For this review, take the finished solid that the model builds, in its own axes (mm). A direction names the side the tool comes from. Coordinates: 2 decimals unless noted, no trailing zeros. Order: outer loops, then holes, each group sorted by start corner. A loop starts at its lowest first (then second) coordinate and runs counter-clockwise, first axis right, second up.
from build123d import *

# Parameters (mm, degrees)
SKETCH1_R          = 8.5
SKETCH1_R_2        = 1.5
BASE_FLANGE1_DEPTH = 3


# Sheet-metal steps are written as plain solids
with BuildPart() as part:
    # Sketch1 → Base-Flange1 (new body)
    with BuildSketch(Plane(origin=(0, 0, 0), x_dir=(1, 0, 0), z_dir=(0, 1, 0))):
        with BuildLine():
            Line((19.609421573, -14.059417906), (10.862109445, -29.480175346))
            ThreePointArc((10.862109445, -29.480175346), (9.762567662, -30.59234701), (8.252687872, -31))
            Line((8.252687872, -31), (-8.352599575, -31))
            ThreePointArc((-8.352599575, -31), (-9.796606082, -30.629609326), (-10.884048227, -29.609896806))
            Line((-10.884048227, -29.609896806), (-20.742852548, -14.107625594))
            ThreePointArc((-20.742852548, -14.107625594), (-21.091885276, -13.336076582), (-21.211403896, -12.497728788))
            Line((-21.211403896, -12.497728788), (-21.211403896, 14.839305313))
            ThreePointArc((-21.211403896, 14.839305313), (-21.044943633, 15.824725306), (-20.564035521, 16.700789784))
            Line((-20.564035521, 16.700789784), (-10.150833328, 29.861484472))
            ThreePointArc((-10.150833328, 29.861484472), (-9.105019706, 30.700412322), (-7.798201703, 31))
            Line((-7.798201703, 31), (7.702138241, 31))
            ThreePointArc((7.702138241, 31), (9.077698333, 30.666052219), (10.147014932, 29.738556288))
            Line((10.147014932, 29.738556288), (19.444876691, 16.663267527))
            ThreePointArc((19.444876691, 16.663267527), (19.857851472, 15.837226972), (20, 14.924711239))
            Line((20, 14.924711239), (20, -12.57924256))
            ThreePointArc((20, -12.57924256), (19.900712388, -13.344662472), (19.609421573, -14.059417906))
        make_face()
        with Locations(Location((7.5, -13.4, 0), (0, 0, 270))):
            Circle(SKETCH1_R, mode=Mode.SUBTRACT)
        with Locations(Location((6, -27, 0), (0, 0, 270))):
            Circle(SKETCH1_R_2, mode=Mode.SUBTRACT)
        with Locations(Location((-6, -27, 0), (0, 0, 270))):
            Circle(SKETCH1_R_2, mode=Mode.SUBTRACT)
        with Locations(Location((5.25, 27.940782939, 0), (0, 0, 270))):
            Circle(SKETCH1_R_2, mode=Mode.SUBTRACT)
        with Locations(Location((-5.25, 27.940782939, 0), (0, 0, 270))):
            Circle(SKETCH1_R_2, mode=Mode.SUBTRACT)
        with Locations(Location((13.5, 7.05, 0), (0, 0, 270))):
            Circle(SKETCH1_R_2, mode=Mode.SUBTRACT)
        with Locations(Location((-13.5, 7.05, 0), (0, 0, 270))):
            Circle(SKETCH1_R_2, mode=Mode.SUBTRACT)
        with BuildLine():
            Line((-13.281403896, 0), (-13.281403896, 1.567980996))
            ThreePointArc((-13.281403896, 1.567980996), (-10.106558233, 2.738982767), (-8.222660082, 5.55))
            Line((-8.222660082, 5.55), (8.208497378, 5.55))
            ThreePointArc((8.208497378, 5.55), (10.031018679, 2.781959631), (13.113110627, 1.563624456))
            ThreePointArc((13.113110627, 1.563624456), (14.07117407, -0.953003234), (11.655254401, -2.142386538))
            ThreePointArc((11.655254401, -2.142386538), (0.639353267, -3.554619032), (-4.5, -13.4))
            ThreePointArc((-4.5, -13.4), (-8.890701948, -17.790701948), (-13.281403896, -13.4))
            Line((-13.281403896, -13.4), (-13.281403896, 0))
        make_face(mode=Mode.SUBTRACT)
        with BuildLine():
            Line((-8.222660082, 8.55), (8.208497378, 8.55))
            ThreePointArc((8.208497378, 8.55), (9.751572067, 11.074833914), (12.37962963, 12.434679214))
            ThreePointArc((12.37962963, 12.434679214), (-0.006957749, 20.549998207), (-12.385173459, 12.42191571))
            ThreePointArc((-12.385173459, 12.42191571), (-9.763306163, 11.067142739), (-8.222660082, 8.55))
        make_face(mode=Mode.SUBTRACT)
    extrude(amount=BASE_FLANGE1_DEPTH)


solid = part.part
1. To check wall thickness, follow L1, parallel to X at y = 1.6, z = -7.05; L2, parallel to X at y = 2.3, z = 27; L3, parallel to Z at x = -6.5, y = 2.3. State the ranges of each line that lie inside material, in increasing order.
Answer below:
L1: x = -21.21 to -15, -12 to 12, 15 to 20
L2: x = -12.54 to -7.5, -4.5 to 4.5, 7.5 to 12.27
L3: z = -31 to -28.77, -27.11 to -18.88, -8.55 to -5.55, 17.08 to 25.59, 28.41 to 31
2. Take a section at B-B, the plane x = -2. Give the boundary of the cut face in (y, z), plus the area to 3 significant figures.
Answer below:
outline: (0, -31) - (3, -31) - (3, -20.4) - (0, -20.4) - close; (0, -8.55) - (3, -8.55) - (3, -5.55) - (0, -5.55) - close; (0, 6.07) - (3, 6.07) - (3, 31) - (0, 31) - close
area: 116 mm2
3. Clearance check with flat-ended pins moving along their axes: pin 1 Ø2.5 at (x, z) = (-6, 27) entering from +Y; pin 2 Ø1 at (x, y) = (-9.5, 0.5) entering from -Z. State where each tip first meets the part, or that it passes through.
Answer below:
pin 1: passes through
pin 2: stops at z = -30.75
4. The part is to be moulded in two halves that separate along Z. For faces 1 (the face through (9.78, 1.48, 30.58)), 2 (the face through (-5.93, 1.48, 25.5)), 3 (the face through (-21.05, 1.48, -15.81)), say which applies: +Z half, -Z half, draft (parallel to the pull), parting line (faces both ways), or undercut.
Answer below:
face 1: +Z half
face 2: undercut
face 3: -Z half
5. Take a section at A-A, the plane z = -7.05. Give the boundary of the cut face in (x, y), plus the area to 3 significant figures.
Answer below:
outline: (-21.21, 0) - (-15, 0) - (-15, 3) - (-21.21, 3) - close; (-12, 0) - (12, 0) - (12, 3) - (-12, 3) - close; (15, 0) - (20, 0) - (20, 3) - (15, 3) - close
area: 106 mm2
6. Take a section at C-C, the plane z = 3. Give the boundary of the cut face in (x, y), plus the area to 4 significant figures.
Answer below:
outline: (-21.21, 0) - (-13.28, 0) - (-13.28, 3) - (-21.21, 3) - close; (1.51, 0) - (20, 0) - (20, 3) - (1.51, 3) - close
area: 79.25 mm2
7. Machinability: for faces 4 (the face through (-15.43, 1.48, -23.19)), 5 (the face through (-13.281, 1, 6)), which of the approach directions +Z, -Z, +X, -X, +Y, -Y give a long, thin tool a straight path to every point of the face, cutting with its end or side? Answer none if there is none.
Answer below:
face 4: -Z, -X, +Y, -Y
face 5: +Y, -Y
8. Take a section at D-D, the plane x = 5.25. Give the boundary of the cut face in (y, z).
Answer below:
outline: (0, -31) - (3, -31) - (3, -29.44) - (0, -29.44) - close; (0, -26.44) - (3, -26.44) - (3, -19.49) - (0, -19.49) - close; (0, -8.55) - (3, -8.55) - (3, -5.55) - (0, -5.55) - close; (0, 1.61) - (3, 1.61) - (3, 5.2) - (0, 5.2) - close; (0, 21.6) - (3, 21.6) - (3, 25.7) - (0, 25.7) - close; (0, 28.3) - (3, 28.3) - (3, 31) - (0, 31) - close
